from build123d import *

# Parameters (mm, degrees)
BOSS_EXTRUDE1_DEPTH        = 44
F_21_0_21_DIAMETER_HOLE1_D = 21
F_26_0_26_DIAMETER_HOLE1_D = 26
BOSS_EXTRUDE2_START        = -1.5
SKETCH9_R                  = 10.5
SKETCH9_R_2                = 8.75
BOSS_EXTRUDE2_DEPTH        = 1.5
BOSS_EXTRUDE3_START        = 88
SKETCH9_2_R                = 10.5
SKETCH9_2_R_2              = 8.75
BOSS_EXTRUDE3_DEPTH        = 1.5
SKETCH16_R                 = 13
SKETCH16_R_2               = 11.25
BOSS_EXTRUDE4_DEPTH        = 1.5
SKETCH17_W                 = 18.25
SKETCH17_H                 = 1.5
CUT_EXTRUDE1_DEPTH         = 80.504716841
CUT_EXTRUDE3_DEPTH         = 121.137421314
FILLET3_R                  = 5
RIB1_REACH                 = 71.778
SKETCH20_WALL_W            = 152.870148694
SKETCH20_WALL_H            = 20
RIB2_REACH                 = 71.778
SKETCH21_WALL_W            = 152.870148694
SKETCH21_WALL_H            = 20
SKETCH22_W                 = 20
SKETCH22_H                 = 38
CUT_EXTRUDE4_DEPTH         = 6
CUT_EXTRUDE5_DEPTH         = 121.137421314
CUT_EXTRUDE5_DEPTH_BACK    = 6
CUT_EXTRUDE6_START         = -104
CUT_EXTRUDE6_DEPTH         = 6
FILLET4_R                  = 4
CHAMFER1_SIZE              = 2


with BuildPart() as part:
    # Sketch1 → Boss-Extrude1 (new body)
    with BuildSketch(Plane.XY):
        Polygon((44, 0), (-44, 0), (-44, -41), (-52, -41), (-52, 8), (52, 8), (52, -41), (44, -41), align=None)
    extrude(amount=BOSS_EXTRUDE1_DEPTH)

    # Ø21.0 (21) Diameter Hole1 (through all)
    with Locations(Plane.ZY.offset(52)):
        with Locations((22, -27)):
            Hole(F_21_0_21_DIAMETER_HOLE1_D / 2)

    # Ø26.0 (26) Diameter Hole1 (through all)
    with Locations(Plane(origin=(0, 8, 0), x_dir=(1, 0, 0), z_dir=(0, 1, 0))):
        with Locations((0, -22)):
            Hole(F_26_0_26_DIAMETER_HOLE1_D / 2)

    # Sketch9 → Boss-Extrude2 (add)
    with BuildSketch(Plane.ZY.offset(-44).offset(BOSS_EXTRUDE2_START)):
        with Locations((22, -27)):
            Circle(SKETCH9_R)
        with Locations((22, -27)):
            Circle(SKETCH9_R_2, mode=Mode.SUBTRACT)
    extrude(amount=BOSS_EXTRUDE2_DEPTH)

    # Sketch9<2> → Boss-Extrude3 (add)
    with BuildSketch(Plane.ZY.offset(-44).offset(BOSS_EXTRUDE3_START)):
        with Locations((22, -27)):
            Circle(SKETCH9_2_R)
        with Locations((22, -27)):
            Circle(SKETCH9_2_R_2, mode=Mode.SUBTRACT)
    extrude(amount=BOSS_EXTRUDE3_DEPTH)

    # Sketch16 → Boss-Extrude4 (add)
    with BuildSketch(Plane(origin=(0, 0, 0), x_dir=(1, 0, 0), z_dir=(0, 1, 0))):
        with Locations(Location((0, -22, 0), (0, 0, 270))):
            Circle(SKETCH16_R)
        with Locations(Location((0, -22, 0), (0, 0, 270))):
            Circle(SKETCH16_R_2, mode=Mode.SUBTRACT)
    extrude(amount=BOSS_EXTRUDE4_DEPTH)

    # Sketch17 → Cut-Extrude1 (cut, through all)
    with BuildSketch(Plane.XY.offset(44)):
        with Locations((0, 0.75)):
            Rectangle(SKETCH17_W, SKETCH17_H)
    extrude(amount=-CUT_EXTRUDE1_DEPTH, mode=Mode.SUBTRACT)

    # Sketch19 → Cut-Extrude3 (cut, through all)
    with BuildSketch(Plane.ZY.offset(52)):
        with BuildLine():
            ThreePointArc((0, -25), (2.087839834, -24.722753708), (4.030968204, -23.910231207))
            Line((4.030968204, -23.910231207), (0, -17))
            Line((0, -17), (0, -25))
        make_face()
        with BuildLine():
            Line((0, -17), (4.030968204, -23.910231207))
            ThreePointArc((4.030968204, -23.910231207), (6.937137221, -20.984485812), (8, -17))
            ThreePointArc((8, -17), (5.656854249, -11.343145751), (0, -9))
            Line((0, -9), (0, -17))
        make_face()
        with BuildLine():
            Line((14, -41), (8, -30.714285714))
            Line((8, -30.714285714), (4.030968204, -23.910231207))
            ThreePointArc((4.030968204, -23.910231207), (2.087839834, -24.722753708), (0, -25))
            Line((0, -25), (0, -41))
            Line((0, -41), (14, -41))
        make_face()
        with BuildLine():
            Line((4.030968204, -23.910231207), (8, -30.714285714))
            Line((8, -30.714285714), (8, -17))
            ThreePointArc((8, -17), (6.937137221, -20.984485812), (4.030968204, -23.910231207))
        make_face()
        with BuildLine():
            Line((36, -17), (36, -30.714285714))
            Line((36, -30.714285714), (39.969031796, -23.910231207))
            ThreePointArc((39.969031796, -23.910231207), (37.062862779, -20.984485812), (36, -17))
        make_face()
        with BuildLine():
            ThreePointArc((39.969031796, -23.910231207), (41.912160166, -24.722753708), (44, -25))
            Line((44, -25), (44, -17))
            Line((44, -17), (39.969031796, -23.910231207))
        make_face()
        with BuildLine():
            ThreePointArc((44, -9), (38.343145751, -11.343145751), (36, -17))
            ThreePointArc((36, -17), (37.062862779, -20.984485812), (39.969031796, -23.910231207))
            Line((39.969031796, -23.910231207), (44, -17))
            Line((44, -17), (44, -9))
        make_face()
        with BuildLine():
            Line((36, -30.714285714), (30, -41))
            Line((30, -41), (44, -41))
            Line((44, -41), (44, -25))
            ThreePointArc((44, -25), (41.912160166, -24.722753708), (39.969031796, -23.910231207))
            Line((39.969031796, -23.910231207), (36, -30.714285714))
        make_face()
    extrude(amount=-CUT_EXTRUDE3_DEPTH, mode=Mode.SUBTRACT)

    # Fillet3
    fillet3_edges = [part.edges().sort_by_distance(p)[0] for p in [
        (48, -9, 0),
        (-48, -9, 0),
        (-48, -9, 44),
        (48, -9, 44),
        (-48, -30.714285714, 36),
        (48, -30.714285714, 36),
        (-48, -41, 30),
        (48, -41, 30),
        (-48, -30.714285714, 8),
        (48, -30.714285714, 8),
        (-48, -41, 14),
        (48, -41, 14),
    ]]
    fillet(fillet3_edges, radius=FILLET3_R)

    # Sketch20 wall → Rib1 (add, up to next)
    with BuildSketch(Plane(origin=(-40, -4, 22), x_dir=(-0.707106781187, -0.707106781187, 0), z_dir=(0.707106781187, -0.707106781187, 0)), mode=Mode.PRIVATE) as rib1_sk1:
        Rectangle(SKETCH20_WALL_W, SKETCH20_WALL_H)
    rib1_tool1 = extrude(rib1_sk1.sketch, amount=-RIB1_REACH, mode=Mode.PRIVATE) - part.part
    add(rib1_tool1.solids().sort_by_distance((-40, -4, 22))[0])

    # Sketch21 wall → Rib2 (add, up to next)
    with BuildSketch(Plane(origin=(40, -4, 22), x_dir=(0.707106781187, -0.707106781187, 0), z_dir=(0.707106781187, 0.707106781187, 0)), mode=Mode.PRIVATE) as rib2_sk1:
        Rectangle(SKETCH21_WALL_W, SKETCH21_WALL_H)
    rib2_tool1 = extrude(rib2_sk1.sketch, amount=RIB2_REACH, mode=Mode.PRIVATE) - part.part
    add(rib2_tool1.solids().sort_by_distance((40, -4, 22))[0])

    # Sketch22 → Cut-Extrude4 (cut)
    with BuildSketch(Plane.XZ):
        with Locations((-26, 22)):
            Rectangle(SKETCH22_W, SKETCH22_H)
        with Locations((26, 22)):
            Rectangle(SKETCH22_W, SKETCH22_H)
    extrude(amount=-CUT_EXTRUDE4_DEPTH, mode=Mode.SUBTRACT)

    # Sketch23 → Cut-Extrude5 (cut, two sides: drawn at the far end of the back side and taken through both)
    with BuildSketch(Plane.ZY.offset(52).offset(-CUT_EXTRUDE5_DEPTH_BACK)):
        with BuildLine():
            Line((40, -5), (40, 4))
            Line((40, 4), (4, 4))
            Line((4, 4), (4, -5))
            ThreePointArc((4, -5), (4.167949706, -5.554700196), (4.615384615, -5.923076923))
            ThreePointArc((4.615384615, -5.923076923), (9.846465163, -10.140909405), (11.989973592, -16.509558097))
            ThreePointArc((11.989973592, -16.509558097), (22, -12.5), (32.010026408, -16.509558097))
            ThreePointArc((32.010026408, -16.509558097), (34.153534837, -10.140909405), (39.384615385, -5.923076923))
            ThreePointArc((39.384615385, -5.923076923), (39.832050294, -5.554700196), (40, -5))
        make_face()
    extrude(amount=CUT_EXTRUDE5_DEPTH + CUT_EXTRUDE5_DEPTH_BACK, mode=Mode.SUBTRACT)

    # Sketch23<3> → Cut-Extrude6 (cut)
    with BuildSketch(Plane.ZY.offset(52).offset(CUT_EXTRUDE6_START)):
        with BuildLine():
            Line((40, -5), (40, 4))
            Line((40, 4), (4, 4))
            Line((4, 4), (4, -5))
            ThreePointArc((4, -5), (4.167949706, -5.554700196), (4.615384615, -5.923076923))
            ThreePointArc((4.615384615, -5.923076923), (9.846465163, -10.140909405), (11.989973592, -16.509558097))
            ThreePointArc((11.989973592, -16.509558097), (22, -12.5), (32.010026408, -16.509558097))
            ThreePointArc((32.010026408, -16.509558097), (34.153534837, -10.140909405), (39.384615385, -5.923076923))
            ThreePointArc((39.384615385, -5.923076923), (39.832050294, -5.554700196), (40, -5))
        make_face()
    extrude(amount=CUT_EXTRUDE6_DEPTH, mode=Mode.SUBTRACT)

    # Fillet4
    fillet4_edges = [part.edges().sort_by_distance(p)[0] for p in [
        (-49, -16.509558097, 11.989973592),
        (-49, -16.509558097, 32.010026408),
        (49, -16.509558097, 32.010026408),
        (49, -16.509558097, 11.989973592),
        (49, 4, 4),
        (49, 4, 40),
        (-49, 4, 40),
        (-49, 4, 4),
        (36, 3, 3),
        (-16, 3, 3),
        (36, 3, 41),
        (-16, 3, 41),
        (-36, 3, 3),
        (16, 3, 3),
        (16, 3, 41),
        (-36, 3, 41),
    ]]
    fillet(fillet4_edges, radius=FILLET4_R)

    # Chamfer1
    chamfer1_edges = [part.edges().sort_by_distance(p)[0] for p in [
        (0, 8, 44),
        (0, 8, 0),
    ]]
    chamfer(chamfer1_edges, length=CHAMFER1_SIZE)


solid = part.part
Verification items for the finished model (mm, model axes). A direction names the side the tool comes from. Give positions to 0.01 mm unless a question says otherwise; leave off trailing zeros. Write each loop counter-clockwise with the first axis right and the second up, starting at its lowest first coordinate (ties: lowest second). Pieces come first, ordered by that corner, then holes. Notation, with made-up numbers: M 30,81.25 L 41,81.25 A24 ccw 41,120.25 Z; hole C 41.25,38 d5. An arc over 180 degrees is marked long. Use CSV: the item, a comma, the result in double quotes.
1) Cross-section at A-A (y = -27). Enter the section's corners in (x, z).
Final values:
outline,"M -52,8 L -44,8 L -44,13.25 L -45.5,13.25 L -45.5,11.5 L -52,11.5 Z; M -52,32.5 L -45.5,32.5 L -45.5,30.75 L -44,30.75 L -44,36 L -52,36 Z; M 44,8 L 52,8 L 52,11.5 L 45.5,11.5 L 45.5,13.25 L 44,13.25 Z; M 44,30.75 L 45.5,30.75 L 45.5,32.5 L 52,32.5 L 52,36 L 44,36 Z"
2) Cross-section at C-C (x = 27). Enter the section's corners in (y, z), plus the area to 3 significant figures.
Final values:
outline,"M 0,0 L 6,0 L 8,2 L 8,42 L 6,44 L 0,44 L 0,41 L 6,41 L 6,3 L 0,3 Z"
area,"120 mm²"
3) Access from +Z, -Z, +X, -X, +Y, -Y to the whole of each face (thin tool, end or side, straight path). Record for faces 4 (the face through (45.5, -19, 18)), 5 (the face through (17.203, 3.042, 4.141)), 6 (the face through (-48, -23, 36)), 7 (the face through (-11.25, 0.74, 21.9)).
Final values:
face 4,"+X"
face 5,"-Y"
face 6,"+Z, +X, -X, -Y"
face 7,"+Y, -Y"
4) Cross-section at D-D (z = 22). State how many separate pieces and enclosed holes the cut face has, plus the area to 3 significant figures.
Final values:
separate pieces,"4"
enclosed holes,"0"
area,"586 mm²"
5) Go/stop test with flat-tipped pins: pin 1 Ø1.6 at (y, z) = (1, 8) entering from +X; pin 2 Ø4 at (x, y) = (46.5, -26) entering from +Z; pin 3 Ø4 at (x, y) = (40.5, -3) entering from -Z. Record where each tip stops, or that it passes through.
Final values:
pin 1,"x = 46"
pin 2,"z = 36"
pin 3,"z = 12"
6) Release check for a two-part mould opening along X. For faces 1 (the face through (-45.5, -19, 18)), 2 (the face through (-48, -23, 8)), 3 (the face through (15, 0, 22)) record: released by +X, released by -X, zero draft, split by the parting line, or undercut.
Final values:
face 1,"released by -X"
face 2,"zero draft"
face 3,"undercut"
7) Cross-section at B-B (x = 0). Enter the section's corners in (y, z), plus the area to 3 significant figures.
Final values:
outline,"M 1.5,0 L 6,0 L 8,2 L 8,9 L 1.5,9 Z; M 1.5,35 L 8,35 L 8,42 L 6,44 L 1.5,44 Z"
area,"113 mm²"
8) Material ranges on line 1 along X through (y, z) = (0.5, 36) (3 decimals); line 2 along Y through (x, z) = (50, 22); line 3 along Y through (x, z) = (-45, 22), recorded low to high.
Final values:
line 1,"-46 to -36, -16 to -9.125, 9.125 to 16, 36 to 46"
line 2,"-41 to -37.5, -16.5 to -12.5, 4 to 8"
line 3,"-41 to -35.75, -18.25 to 8"
